from build123d import *

# Parameters (mm, degrees)
F0_R     = 45.631
F0_R_2   = 40.631
F1_DEPTH = 8
F4_SIZE  = 1


with BuildPart() as f1:
    # F0 (on Top) → F1 (new body)
    with BuildSketch(Plane.XY):
        Circle(F0_R)
        Circle(F0_R_2, mode=Mode.SUBTRACT)
    extrude(amount=F1_DEPTH)

    # F2 (on Right) → F3 (revolve)
    with BuildSketch(Plane.YZ):
        Polygon((40.631, 3), (45.631, 3), (36.235, 53.383008), (36.235, 58.383008), (31.235, 58.383008), (31.235, 53.383008), align=None)
    revolve(axis=Axis((0, 0, 34.883008), (0, 0, 1)))

    # F4
    f4_edges = [f1.edges().sort_by_distance(p)[0] for p in [
        (-40.631, 0, 0),
    ]]
    chamfer(f4_edges, length=F4_SIZE)


solid = f1.part
Source: CAD feature listing. Evaluate the final solid. Frame: model axes, mm. A direction names the side the tool comes from. Give positions to 0.01 mm unless a question says otherwise; leave off trailing zeros. Write each loop counter-clockwise with the first axis right and the second up, starting at its lowest first coordinate (ties: lowest second). Pieces come first, ordered by that corner, then holes. Notation, with made-up numbers: M 45,87.25 L 87,87.25 A7 ccw 87,93.25 Z; hole C -10,85 d4. An arc over 180 degrees is marked long. Return JSON: item names as keys, results as strings. Group by question number.
1) Cut plane D-D, the plane z = 43.5. Output: boundary loops of the cut face in (x, y).
2) Cut plane C-C, the plane z = 37. Output: boundary loops of the cut face in (x, y).
3) Set-up query: faces 4 (the face through (-10.884, 34.562, 55.918)), 5 (the face through (38.755, 12.204, 1.986)), 6 (the face through (-30, 11, 58.383)). Return all of +Z, -Z, +X, -X, +Y, -Y with unobstructed straight access to the full face (end or side cutting, diameter ignored); none if empty.
4) Ray query, L1, parallel to Y at x = 0, z = 54 (3 decimals); L2, parallel to Y at x = 0, z = 2. Return the intervals inside material, ascending.
5) First-contact query: pin 1 Ø1.5 at (y, z) = (-27, 27.5) entering from -X; pin 2 Ø8 at (y, z) = (19.5, 51.5) entering from -X; pin 3 Ø10 at (x, z) = (34, 13) entering from -Y. Flat tips, straight axial feed; report the tip coordinate or a pass-through.
6) Draft query along X for faces 1 (the face through (37, -20, 0)), 2 (the face through (38.53, -8.56, 36.05)), 3 (the face through (-9.382, 29.793, 55.848)). Return one class per face: released by +X, released by -X, zero draft, split by the parting line, or undercut.
7) Cut plane A-A, the plane x = 0. Output: boundary loops of the cut face in (y, z) (3 decimals).
Data:
{
 "1": {"outline": "C 0,0 d76.16; hole C 0,0 d66.16"},
 "2": {"outline": "C 0,0 d78.58; hole C 0,0 d68.58"},
 "3": {"face 4": "+Z", "face 5": "-Z", "face 6": "+Z, +X, -X, +Y, -Y"},
 "4": {"L1": "y = -36.235 to -31.235, 31.235 to 36.235", "L2": "y = -45.63 to -40.63, 40.63 to 45.63"},
 "5": {"pin 1": "stops at x = -31.6", "pin 2": "stops at x = -33.31", "pin 3": "stops at y = -32.95"},
 "6": {"face 1": "zero draft", "face 2": "split by the parting line", "face 3": "undercut"},
 "7": {"outline": "M -45.631,0 L -41.631,0 L -40.631,1 L -40.631,3 L -31.235,53.383 L -31.235,58.383 L -36.235,58.383 L -36.235,53.383 L -44.699,8 L -45.631,8 Z; M 31.235,53.383 L 40.631,3 L 40.631,1 L 41.631,0 L 45.631,0 L 45.631,8 L 44.699,8 L 36.235,53.383 L 36.235,58.383 L 31.235,58.383 Z"}
}
